The listing builds one solid part. Answer for the finished solid, in the listing's coordinates (mm). Round coordinates to 2 decimals unless told otherwise and drop trailing zeros. Write each loop counter-clockwise with the first axis right and the second up, starting at its lowest first coordinate (ties: lowest second). Pieces come first, ordered by that corner, then holes.
(1) A cutting plane is placed at B-B, the plane y = -11.4. Give the vertices of the cut face in (x, z) (3 decimals), and give its area (3 significant figures).
(2) A cutting plane is placed at D-D, the plane z = 3.75. Give the vertices of the cut face in (x, y) (1 decimal).
(3) Find the intervals of material crossed by probe 1 along Y at (x, z) = (0.5, 6.75) (3 decimals); probe 2 along X at (y, z) = (-22, 1) (3 decimals); probe 3 along Y at (x, z) = (0, 4.5) (3 decimals), in increasing order.
(4) Each of these flat-tipped pins is pushed along its axis until it touches: pin 1 Ø12.5 at (x, y) = (-65.5, -11.4) entering from -Z; pin 2 Ø4 at (x, y) = (58.5, 185) entering from +Z; pin 3 Ø5 at (x, z) = (-67.5, 3.5) entering from +Y; pin 4 Ø3 at (y, z) = (149.5, 6) entering from -X (3 decimals). Where does it stop, or does it pass through?
(5) A cutting plane is placed at A-A, the plane x = 0. Give the vertices of the cut face in (y, z) (3 decimals), and give its area (3 significant figures).
(6) A cutting plane is placed at C-C, the plane x = -65.5. Give the vertices of the cut face in (y, z).
from build123d import *

# Parameters (mm, degrees)
SKETCH_R       = 3.96875
SKETCH_W       = 116.4
SKETCH_H       = 65.9
PAD_DEPTH      = 10
BOX_W          = 110.05
BOX_H          = 282.45
BOX_DEPTH      = 10
CYLINDER_R     = 3.03
CYLINDER_DEPTH = 10


with BuildPart() as part:
    # Sketch → Pad (new body)
    with BuildSketch(Plane.XY):
        with BuildLine():
            Line((78.2, 0), (-78.2, 0))
            Line((-78.2, 0), (-78.2, -72.9))
            ThreePointArc((-78.2, -72.9), (-77.028427, -75.728427), (-74.2, -76.9))
            Line((-74.2, -76.9), (74.2, -76.9))
            ThreePointArc((74.2, -76.9), (77.028427, -75.728427), (78.2, -72.9))
            Line((78.2, -72.9), (78.2, 0))
        make_face()
        with Locations((-65.5, -11.4)):
            Circle(SKETCH_R, mode=Mode.SUBTRACT)
        with Locations((65.5, -11.4)):
            Circle(SKETCH_R, mode=Mode.SUBTRACT)
        with Locations((0, -33.95)):
            Rectangle(SKETCH_W, SKETCH_H, mode=Mode.SUBTRACT)
    extrude(amount=PAD_DEPTH)

    # Box → Box (join)
    with BuildSketch(Plane(origin=(-55.025, -63.725, 0), x_dir=(1, 0, 0), z_dir=(0, 0, 1))):
        with Locations((55.025, 141.225)):
            Rectangle(BOX_W, BOX_H)
    extrude(amount=BOX_DEPTH)

    # Cylinder → Cylinder (cut)
    with BuildSketch(Plane(origin=(0, -53.725, 0), x_dir=(1, 0, 0), z_dir=(0, 0, 1))):
        Circle(CYLINDER_R)
    extrude(amount=CYLINDER_DEPTH, mode=Mode.SUBTRACT)


solid = part.part
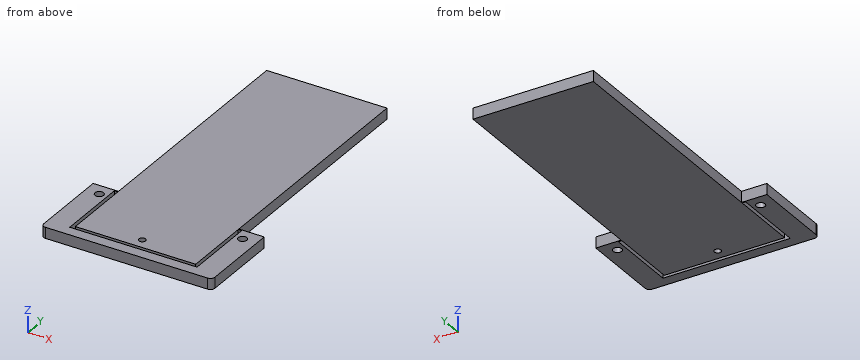
Solutions:
1. outline: (-78.2, 0) - (-69.469, 0) - (-69.469, 10) - (-78.2, 10) - close; (-61.531, 0) - (-58.2, 0) - (-58.2, 10) - (-61.531, 10) - close; (-55.025, 0) - (55.025, 0) - (55.025, 10) - (-55.025, 10) - close; (58.2, 0) - (61.531, 0) - (61.531, 10) - (58.2, 10) - close; (69.469, 0) - (78.2, 0) - (78.2, 10) - (69.469, 10) - close
1. area: 1,340 mm2
2. outline: (-78.2, -72.9) arc R4 ccw to (-74.2, -76.9) - (74.2, -76.9) arc R4 ccw to (78.2, -72.9) - (78.2, 0) - (55, 0) - (55, 218.7) - (-55, 218.7) - (-55, 0) - (-78.2, 0) - close; hole circle Ø7.9 at (-65.5, -11.4); hole (-58.2, -66.9) - (58.2, -66.9) - (58.2, -1) - (55, -1) - (55, -63.7) - (-55, -63.7) - (-55, -1) - (-58.2, -1) - close; hole circle Ø6.1 at (0, -53.7); hole circle Ø7.9 at (65.5, -11.4)
3. probe 1: y = -76.9 to -66.9, -63.725 to -56.713, -50.737 to 218.725
3. probe 2: x = -78.2 to -58.2, -55.025 to 55.025, 58.2 to 78.2
3. probe 3: y = -76.9 to -66.9, -63.725 to -56.755, -50.695 to 218.725
4. pin 1: stops at z = 0
4. pin 2: passes through
4. pin 3: stops at y = 0
4. pin 4: stops at x = -55.025
5. outline: (-76.9, 0) - (-66.9, 0) - (-66.9, 10) - (-76.9, 10) - close; (-63.725, 0) - (-56.755, 0) - (-56.755, 10) - (-63.725, 10) - close; (-50.695, 0) - (218.725, 0) - (218.725, 10) - (-50.695, 10) - close
5. area: 2,860 mm2
6. outline: (-76.9, 0) - (-15.37, 0) - (-15.37, 10) - (-76.9, 10) - close; (-7.43, 0) - (0, 0) - (0, 10) - (-7.43, 10) - close
